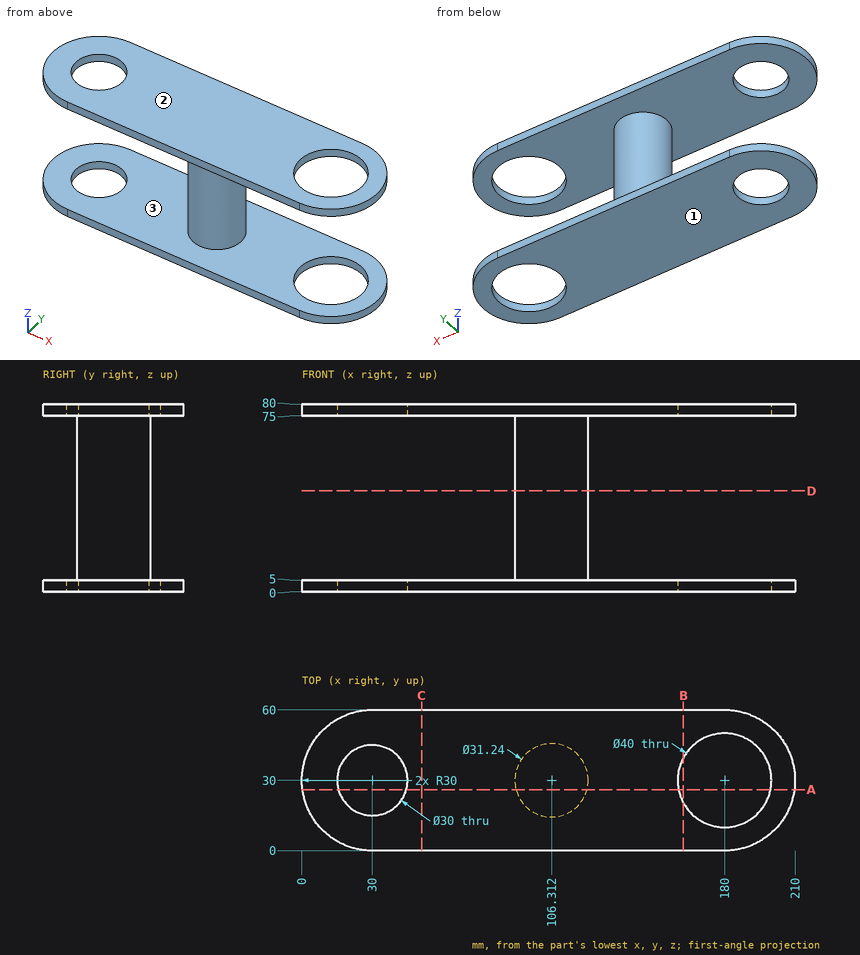
Here's the drawing with two shaded views (mm, measured from the low corner). I have some questions. Coordinates: 2 decimals unless noted, no trailing zeros. Order: outer loops, then holes, each group sorted by start corner. A loop starts at its lowest first (then second) coordinate and runs counter-clockwise, first axis right, second up.
Item 1: If we mould it in two halves opening along Z, with no side actions, what happens to the marked faces 1, 2 and 3? For each: +Z half, -Z half, draft (parallel to the pull), parting line (faces both ways), or undercut.
Result sheet:
face 1: -Z half
face 2: +Z half
face 3: undercut
Item 2: If we section it at C-C on x = 51: List the corners of the cut face in (y, z) for me.
Result sheet:
outline: (0, 0) - (60, 0) - (60, 5) - (0, 5) - close; (0, 75) - (60, 75) - (60, 80) - (0, 80) - close
Item 3: If we section it at B-B on x = 162.5: List the corners of the cut face in (y, z) for me, plus the area to 3 significant figures.
Result sheet:
outline: (0, 0) - (20.32, 0) - (20.32, 5) - (0, 5) - close; (0, 75) - (20.32, 75) - (20.32, 80) - (0, 80) - close; (39.68, 0) - (60, 0) - (60, 5) - (39.68, 5) - close; (39.68, 75) - (60, 75) - (60, 80) - (39.68, 80) - close
area: 406 mm2
Item 4: If we section it at D-D on z = 43: List the corners of the cut face in (x, y) for me.
Result sheet:
outline: circle Ø31.24 at (106.31, 30)
Item 5: I need wall thicknesses on line 1 (Y direction, x = 30, z = 3.45); line 2 (Z direction, x = 199.5, y = 8); line 3 (Y direction, x = 180, z = 78). Which ranges of each line are inside material? Lowest first, please.
Result sheet:
line 1: y = 0 to 15, 45 to 60
line 2: z = 0 to 5, 75 to 80
line 3: y = 0 to 10, 50 to 60
Item 6: For P1, Ø8, axis at x = 119.5, z = 31.5, coming from the -Y side; P2, Ø2, axis at y = 20, z = 52, coming from the -X side; P3, Ø3, axis at y = 44.5, z = 59.5, coming from the +X side, each with a flat end and sliding along its axis, tell me the tip position at first contact or that it passes through.
Result sheet:
P1: stops at y = 17.37
P2: stops at x = 93.55
P3: stops at x = 114.97
Item 7: If we section it at A-A on y = 26: List the corners of the cut face in (x, z) for me.
Result sheet:
outline: (0.27, 0) - (15.54, 0) - (15.54, 5) - (0.27, 5) - close; (0.27, 75) - (15.54, 75) - (15.54, 80) - (0.27, 80) - close; (44.46, 0) - (160.4, 0) - (160.4, 5) - (121.41, 5) - (121.41, 75) - (160.4, 75) - (160.4, 80) - (44.46, 80) - (44.46, 75) - (91.21, 75) - (91.21, 5) - (44.46, 5) - close; (199.6, 0) - (209.73, 0) - (209.73, 5) - (199.6, 5) - close; (199.6, 75) - (209.73, 75) - (209.73, 80) - (199.6, 80) - close
